```python
from build123d import *

# Parameters (mm, degrees)
F1_DEPTH = 107.95
F2_DEPTH = 158.75
F4_DEPTH = 2
F5_DEPTH = 2
F6_DEPTH = 2
F7_DEPTH = 2


with BuildPart() as f1:
    # F0 (on Right) → F1 (new body, symmetric)
    with BuildSketch(Plane.YZ):
        with BuildLine():
            ThreePointArc((-10, 0), (-7.0710678119, 7.0710678119), (0, 10))
            Line((0, 10), (-10, 10))
            Line((-10, 10), (-10, 0))
        make_face()
    extrude(amount=F1_DEPTH, both=True)


with BuildPart() as f1b:
    # F0 (on Right) → F1, piece 2 (new body, symmetric)
    with BuildSketch(Plane.YZ):
        with BuildLine():
            ThreePointArc((0, 10), (7.0710678119, 7.0710678119), (10, 0))
            Line((10, 0), (10, 10))
            Line((10, 10), (0, 10))
        make_face()
    extrude(amount=F1_DEPTH, both=True)


with BuildPart() as f1c:
    # F0 (on Right) → F1, piece 3 (new body, symmetric)
    with BuildSketch(Plane.YZ):
        with BuildLine():
            Line((10, -10), (10, 0))
            ThreePointArc((10, 0), (7.0710678119, -7.0710678119), (0, -10))
            Line((0, -10), (10, -10))
        make_face()
    extrude(amount=F1_DEPTH, both=True)


with BuildPart() as f1d:
    # F0 (on Right) → F1, piece 4 (new body, symmetric)
    with BuildSketch(Plane.YZ):
        with BuildLine():
            Line((-10, -10), (0, -10))
            ThreePointArc((0, -10), (-7.0710678119, -7.0710678119), (-10, 0))
            Line((-10, 0), (-10, -10))
        make_face()
    extrude(amount=F1_DEPTH, both=True)


with BuildPart() as f2:
    # F0 (on Right) → F2 (new body, symmetric)
    with BuildSketch(Plane.YZ):
        with BuildLine():
            ThreePointArc((0, -10), (7.0710678119, -7.0710678119), (10, 0))
            ThreePointArc((10, 0), (7.0710678119, 7.0710678119), (0, 10))
            ThreePointArc((0, 10), (-7.0710678119, 7.0710678119), (-10, 0))
            ThreePointArc((-10, 0), (-7.0710678119, -7.0710678119), (0, -10))
        make_face()
    extrude(amount=F2_DEPTH, both=True)


with BuildPart() as f1_1:
    add(f1.part)

    # F3: union F1b, F2, F1c, F1d
    add(f1b.part)
    add(f2.part)
    add(f1c.part)
    add(f1d.part)

    # F4 (add): a face of the model
    f4_faces = [f1_1.faces().sort_by_distance(p)[0] for p in [
        (0, 0, 10),
    ]]
    extrude(f4_faces, amount=F4_DEPTH)

    # F5 (add): a face of the model
    f5_faces = [f1_1.faces().sort_by_distance(p)[0] for p in [
        (0, -10, 1),
    ]]
    extrude(f5_faces, amount=F5_DEPTH)

    # F6 (add): a face of the model
    f6_faces = [f1_1.faces().sort_by_distance(p)[0] for p in [
        (0, 10, 1),
    ]]
    extrude(f6_faces, amount=F6_DEPTH)

    # F7 (add): a face of the model
    f7_faces = [f1_1.faces().sort_by_distance(p)[0] for p in [
        (0, 0, -10),
    ]]
    extrude(f7_faces, amount=F7_DEPTH)


solid = f1_1.part
```
Source: CAD feature listing. Evaluate the final solid. Frame: model axes, mm. A direction names the side the tool comes from. Round coordinates to 2 decimals unless told otherwise and drop trailing zeros. Loops run counter-clockwise (first coordinate to the right, second up) from the corner with the lowest first, then second, coordinate; pieces in that order, holes last. Notation, with made-up numbers: M -2,-10.75 L 39,-10.75 A31 cw 39,25.25 Z; hole C -23.5,9 d2. An arc over 180 degrees is marked long. Use a Markdown table: item, result. Add a question column.
1. Section query B-B on z = -3. Return the cut outline in (x, y), then the cut area to 3 significant figures.
2. Reachability of faces 1 (the flat face through (107.95, 10.5, 0.2)), 2 (the flat face through (2, -12, 0)), 3 (the flat face through (-107.95, 10.5, 0.2)) from +Z, -Z, +X, -X, +Y, -Y: full face, straight path, thin tool, end or side. Return the list, or none.
3. Line query: line 1 (Y direction, x = 131, z = -0.5); line 2 (X direction, y = -10.5, z = -2.5); line 3 (Y direction, x = -138, z = -9). Output: solid intervals per line, ascending.
4. Section query C-C on x = 111.5. Return the cut outline in (y, z).
5. Section query A-A on y = -5. Return the cut outline in (x, z), then the cut area to 3 significant figures.
Reported:
| question | item | result |
|---|---|---|
| 1 | outline | M -158.75,-9.54 L -107.95,-9.54 L -107.95,-12 L 107.95,-12 L 107.95,-9.54 L 158.75,-9.54 L 158.75,9.54 L 107.95,9.54 L 107.95,12 L -107.95,12 L -107.95,9.54 L -158.75,9.54 Z |
| 1 | area | 7,120 mm² |
| 2 | face 1 | +X |
| 2 | face 2 | +Z, -Z, +X, -X, -Y |
| 2 | face 3 | -X |
| 3 | line 1 | y = -9.99 to 9.99 |
| 3 | line 2 | x = -107.95 to 107.95 |
| 3 | line 3 | y = -4.36 to 4.36 |
| 4 | outline | C 0,0 d20 |
| 5 | outline | M -158.75,-8.66 L -107.95,-8.66 L -107.95,-12 L 107.95,-12 L 107.95,-8.66 L 158.75,-8.66 L 158.75,8.66 L 107.95,8.66 L 107.95,12 L -107.95,12 L -107.95,8.66 L -158.75,8.66 Z |
| 5 | area | 6,940 mm² |
